Autodesk Inventor part; units mm, degrees
ref_plane "YZ Plane" through (0, 0, 0) normal (1, 0, 0) x (0, 1, 0)
ref_plane "XZ Plane" through (0, 0, 0) normal (0, 1, 0) x (-1, 0, 0)
ref_plane "XY Plane" through (0, 0, 0) normal (0, 0, 1) x (1, 0, 0)
sketch "Эскиз1" plane through (0, 0, 0) normal (0, 1, 0) x (-1, 0, 0)
  line L0 (21.1, -21.1) -> (-21.1, -21.1)
  line L1 (-21.1, -21.1) -> (-21.1, 21.1)
  line L2 (-21.1, 21.1) -> (21.1, 21.1)
  line L3 (21.1, 21.1) -> (21.1, -21.1)
  line L4 (21.1, -21.1) -> (-21.1, 21.1) construction
  line L5 (-21.1, -21.1) -> (21.1, 21.1) construction
  line L6 (-15.55, 15.55) -> (15.55, 15.55) construction
  line L7 (15.55, 15.55) -> (15.55, -15.55) construction
  line L8 (15.55, -15.55) -> (-15.55, -15.55) construction
  line L9 (-15.55, -15.55) -> (-15.55, 15.55) construction
  line L10 (-15.55, 15.55) -> (15.55, -15.55) construction
  line L11 (15.55, 15.55) -> (-15.55, -15.55) construction
  circle A0 centre (-15.55, -15.55) radius 1.5
  circle A1 centre (15.55, -15.55) radius 1.5
  circle A2 centre (15.55, 15.55) radius 1.5
  circle A3 centre (-15.55, 15.55) radius 1.5
  point P0 (0, 0)
  dimension "d0" = 42.2
  dimension "d1" = 42.2
  dimension "d2" = 31.1
  dimension "d3" = 31.1
  dimension "d4" = 3
  dimension "d5" = 3
  dimension "d6" = 3
  dimension "d7" = 3
extrude "Выдавливание1" add sketch "Эскиз1" along normal blind 8
chamfer "Фаска1" distance 4.5 angle 45 4 edges at (21.1, 4, -21.1) (21.1, 4, 21.1) (-21.1, 4, 21.1) (-21.1, 4, -21.1)
thread "Резьба1"
thread "Резьба2"
thread "Резьба3"
thread "Резьба4"
properties part number "Top"
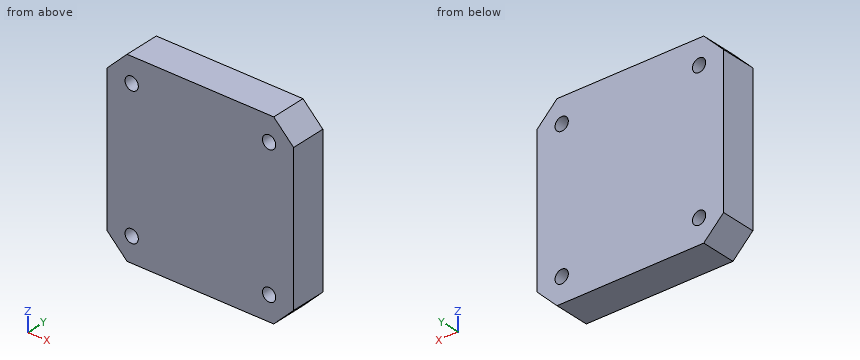
Part model, mm, in its own coordinate system. Coordinates: 2 decimals unless noted, no trailing zeros. Order: outer loops, then holes, each group sorted by start corner. A loop starts at its lowest first (then second) coordinate and runs counter-clockwise, first axis right, second up. Notation, with made-up numbers: M 47.25,78 L 104.25,78 A25 ccw 104.25,113 Z; hole C -25,-33.75 d10. An arc over 180 degrees is marked long. Use a Markdown table: item, result.
(1) Probe L1, parallel to Z at x = 15.55, y = 3.5; L2, parallel to X at y = 0.5, z = 14.5. List the from-to ranges inside material, lowest first.
A:
| item | result |
|---|---|
| L1 | z = -21.1 to -17.05, -14.05 to 14.05, 17.05 to 21.1 |
| L2 | x = -21.1 to -16.62, -14.48 to 14.48, 16.62 to 21.1 |
(2) Cut at A-A on x = 15.55. Write the cut outline in (y, z).
A:
| item | result |
|---|---|
| outline | M 0,-21.1 L 8,-21.1 L 8,-17.05 L 0,-17.05 Z; M 0,-14.05 L 8,-14.05 L 8,14.05 L 0,14.05 Z; M 0,17.05 L 8,17.05 L 8,21.1 L 0,21.1 Z |
(3) Cut at B-B on z = 15.55. Write the cut outline in (x, y).
A:
| item | result |
|---|---|
| outline | M -21.1,0 L -17.05,0 L -17.05,8 L -21.1,8 Z; M -14.05,0 L 14.05,0 L 14.05,8 L -14.05,8 Z; M 17.05,0 L 21.1,0 L 21.1,8 L 17.05,8 Z |
(4) Cut at C-C on y = 2.25. Write the cut outline in (x, z).
A:
| item | result |
|---|---|
| outline | M -21.1,-16.6 L -16.6,-21.1 L 16.6,-21.1 L 21.1,-16.6 L 21.1,16.6 L 16.6,21.1 L -16.6,21.1 L -21.1,16.6 Z; hole C -15.55,-15.55 d3; hole C -15.55,15.55 d3; hole C 15.55,-15.55 d3; hole C 15.55,15.55 d3 |
(5) Flat gauge pin, fed straight in: pin 1 (2.5 mm diameter, centred on x = -15.55, z = 15.55, fed in from -Y). Where does the tip first touch, or does it go through?
A:
| item | result |
|---|---|
| pin 1 | passes through |
